```python
from build123d import *

# Parameters (mm, degrees)
SKETCH1_W           = 77
SKETCH1_H           = 14
BOSS_EXTRUDE1_DEPTH = 2
SKETCH3_W           = 9
SKETCH3_H           = 2
BOSS_EXTRUDE2_DEPTH = 10.8
SKETCH4_W           = 9
SKETCH4_H           = 2
BOSS_EXTRUDE3_DEPTH = 10.8
SKETCH5_W           = 10.8
SKETCH5_H           = 9
BOSS_EXTRUDE4_DEPTH = 6.5
SKETCH6_W           = 8.16
SKETCH6_H           = 3
SKETCH6_W_2         = 7.44
CUT_EXTRUDE1_DEPTH  = 9
SKETCH8_R           = 1.5
CUT_EXTRUDE2_DEPTH  = 8.5
SKETCH10_W          = 9.3
SKETCH10_H          = 6
CUT_EXTRUDE4_DEPTH  = 2
CHAMFER1_SIZE       = 9
CHAMFER1_SIZE2      = 2
BOSS_EXTRUDE5_DEPTH = 5
SKETCH13_R          = 4
CUT_EXTRUDE5_DEPTH  = 5
FILLET3_R           = 1


with BuildPart() as part:
    # Sketch1 → Boss-Extrude1 (new body)
    with BuildSketch(Plane(origin=(0, 0, 0), x_dir=(1, 0, 0), z_dir=(0, 1, 0))):
        with Locations((-53.253755964, -5.729579977)):
            Rectangle(SKETCH1_W, SKETCH1_H)
    extrude(amount=BOSS_EXTRUDE1_DEPTH)

    # Sketch3 → Boss-Extrude2 (add)
    with BuildSketch(Plane.ZY.offset(91.753755964)):
        with Locations((5.729579977, 1)):
            Rectangle(SKETCH3_W, SKETCH3_H)
    extrude(amount=BOSS_EXTRUDE2_DEPTH)

    # Sketch4 → Boss-Extrude3 (add)
    with BuildSketch(Plane(origin=(-14.753755964, 0, 0), x_dir=(0, 0, -1), z_dir=(1, 0, 0))):
        with Locations((-5.729579977, 1)):
            Rectangle(SKETCH4_W, SKETCH4_H)
    extrude(amount=BOSS_EXTRUDE3_DEPTH)

    # Sketch5 → Boss-Extrude4 (add)
    with BuildSketch(Plane(origin=(0, 2, 0), x_dir=(1, 0, 0), z_dir=(0, 1, 0))):
        with Locations((-97.153755964, -5.729579977)):
            Rectangle(SKETCH5_W, SKETCH5_H)
        with Locations((-9.353755964, -5.729579977)):
            Rectangle(SKETCH5_W, SKETCH5_H)
    extrude(amount=BOSS_EXTRUDE4_DEPTH)

    # Sketch6 → Cut-Extrude1 (cut)
    with BuildSketch(Plane.XY.offset(10.229579977)):
        with Locations((-9.353755964, 5.25)):
            Rectangle(SKETCH6_W, SKETCH6_H)
        with Locations((-97.153755964, 5.25)):
            Rectangle(SKETCH6_W_2, SKETCH6_H)
    extrude(amount=-CUT_EXTRUDE1_DEPTH, mode=Mode.SUBTRACT)

    # Sketch8 → Cut-Extrude2 (cut)
    with BuildSketch(Plane(origin=(0, 8.5, 0), x_dir=(1, 0, 0), z_dir=(0, 1, 0))):
        with Locations((-88.178755964, -9.379579977)):
            Circle(SKETCH8_R)
        with Locations((-18.328755964, -9.379579977)):
            Circle(SKETCH8_R)
        with Locations((-97.003755964, -5.729579977)):
            Circle(SKETCH8_R)
        with Locations((-9.503755964, -5.729579977)):
            Circle(SKETCH8_R)
    extrude(amount=-CUT_EXTRUDE2_DEPTH, mode=Mode.SUBTRACT)

    # Sketch10 → Cut-Extrude4 (cut)
    with BuildSketch(Plane(origin=(0, 0, 0), x_dir=(-1, 0, 0), z_dir=(0, -1, 0))):
        with Locations((97.903755964, -5.729579977)):
            Rectangle(SKETCH10_W, SKETCH10_H)
        with Locations((8.603755964, -5.729579977)):
            Rectangle(SKETCH10_W, SKETCH10_H)
    extrude(amount=-CUT_EXTRUDE4_DEPTH, mode=Mode.SUBTRACT)

    # Chamfer1
    chamfer1_edges = [part.edges().sort_by_distance(p)[0] for p in [
        (-102.553755964, 0, 1.979579977),
        (-3.953755964, 0, 9.479579977),
        (-3.953755964, 0, 1.979579977),
        (-102.553755964, 0, 9.479579977),
    ]]
    chamfer1_side = [part.faces().sort_by_distance(p)[0] for p in [
        (-53.253755964, 0, 5.684579251),
    ]]
    chamfer(chamfer1_edges, length=CHAMFER1_SIZE, length2=CHAMFER1_SIZE2, reference=chamfer1_side[0])

    # Sketch12 → Boss-Extrude5 (add)
    with BuildSketch(Plane(origin=(0, 2, 0), x_dir=(1, 0, 0), z_dir=(0, 1, 0))):
        with BuildLine():
            Line((-26.753755964, -12.729579977), (-14.753755964, -12.729579977))
            Line((-14.753755964, -12.729579977), (-14.753755964, -18.729579977))
            ThreePointArc((-14.753755964, -18.729579977), (-20.753755964, -24.729579977), (-26.753755964, -18.729579977))
            Line((-26.753755964, -18.729579977), (-26.753755964, -12.729579977))
        make_face()
        with BuildLine():
            Line((-91.753755964, -12.729579977), (-91.753755964, -18.729579977))
            ThreePointArc((-91.753755964, -18.729579977), (-85.753755964, -24.729579977), (-79.753755964, -18.729579977))
            Line((-79.753755964, -18.729579977), (-79.753755964, -12.729579977))
            Line((-79.753755964, -12.729579977), (-91.753755964, -12.729579977))
        make_face()
    extrude(amount=-BOSS_EXTRUDE5_DEPTH)

    # Sketch13 → Cut-Extrude5 (cut)
    with BuildSketch(Plane(origin=(0, 2, 0), x_dir=(1, 0, 0), z_dir=(0, 1, 0))):
        with Locations((-85.753755964, -18.729579977)):
            Circle(SKETCH13_R)
        with Locations((-20.753755964, -18.729579977)):
            Circle(SKETCH13_R)
    extrude(amount=-CUT_EXTRUDE5_DEPTH, mode=Mode.SUBTRACT)

    # Fillet3
    fillet3_edges = [part.edges().sort_by_distance(p)[0] for p in [
        (-85.753755964, -3, 12.729579977),
        (-85.753755964, 2, 24.729579977),
        (-79.753755964, 2, 15.729579977),
        (-20.753755964, -3, 12.729579977),
        (-20.753755964, 2, 24.729579977),
        (-26.753755964, 2, 15.729579977),
        (-91.753755964, 8.5, 5.729579977),
        (-102.553755964, 8.5, 5.729579977),
        (-14.753755964, 8.5, 5.729579977),
        (-3.953755964, 8.5, 5.729579977),
        (-91.753755964, 1, -1.270420023),
        (-14.753755964, 1, -1.270420023),
    ]]
    fillet(fillet3_edges, radius=FILLET3_R)


solid = part.part
```
Can you work these out from the model? Positions are in its coordinate system, mm. A direction names the side the tool comes from. Give positions to 0.01 mm unless a question says otherwise; leave off trailing zeros. Write each loop counter-clockwise with the first axis right and the second up, starting at its lowest first coordinate (ties: lowest second). Pieces come first, ordered by that corner, then holes. Notation, with made-up numbers: (-13, -29.75) -> (-4, -29.75) arc R29 ccw to (-4, -4.75) -> close; hole circle Ø4 at (21.5, 77.5). An arc over 180 degrees is marked (long way). One line per item, written item: value.
Q1. For P1, Ø2, axis at x = -98, z = 7, coming from the -Y side; P2, Ø12, axis at x = -61, z = 9.5, coming from the +Y side; P3, Ø3, axis at x = -29.5, z = 6, coming from the -Y side, each with a flat end and sliding along its axis, tell me the tip position at first contact or that it passes through.
Results found:
P1: stops at y = 2
P2: stops at y = 2
P3: stops at y = 0
Q2. Please list where these lines run through material, in increasing order: line 1 (X direction, y = 4.75, z = 6); line 2 (X direction, y = 3.25, z = 4.5); line 3 (X direction, y = 3, z = 2.25). Write a range as [from, to].
Results found:
line 1: x = [-102.55, -100.87], [-93.43, -91.75], [-14.75, -13.43], [-5.27, -3.95]
line 2: x = [-102.55, -97.86], [-96.14, -91.75], [-14.75, -10.36], [-8.64, -3.95]
line 3: x = [-102.55, -91.75], [-14.75, -3.95]
Q3. Which directions (+Z, -Z, +X, -X, +Y, -Y) give clear straight access to the entire face, cutting with the end or side of a thin tool? Please do faces 5 (the face through (-97, 1, 8.73)), 6 (the face through (-13.254, 1, 6)), 7 (the face through (-26.754, -1, 16)), 8 (the face through (-93.434, 5, 6)), 9 (the face through (-9, 3, 1.23)).
Results found:
face 5: -X, -Y
face 6: +X, -Y
face 7: +Z, +Y, -Y
face 8: +Z, -Z
face 9: -Z, +X, +Y, -Y
Q4. Imagine slicing it at B-B on x = -78.5. Please give me the cut outline in (y, z).
Results found:
outline: (0, -1.27) -> (2, -1.27) -> (2, 12.73) -> (0, 12.73) -> close
Q5. Imagine slicing it at A-A on y = 5.5. Please give me the cut outline in (x, z).
Results found:
outline: (-102.55, 1.23) -> (-100.87, 1.23) -> (-100.87, 10.23) -> (-102.55, 10.23) -> close; (-93.43, 1.23) -> (-91.75, 1.23) -> (-91.75, 10.23) -> (-93.43, 10.23) -> close; (-14.75, 1.23) -> (-13.43, 1.23) -> (-13.43, 10.23) -> (-14.75, 10.23) -> close; (-5.27, 1.23) -> (-3.95, 1.23) -> (-3.95, 10.23) -> (-5.27, 10.23) -> close
Q6. We'd pull the mould along Z, two halves only. Please class faces 1 (the face through (-8.391, 1.014, 9.49)), 2 (the face through (-97, 3, 10.23)), 3 (the face through (-81.938, -0.465, 17.528)), 4 (the face through (-97, 3, 1.23)): +Z half, -Z half, draft (parallel to the pull), parting line (faces both ways), or undercut.
Results found:
face 1: draft
face 2: +Z half
face 3: undercut
face 4: -Z half
